from build123d import *

# Parameters (mm, degrees)
F0_W     = 70
F0_H     = 70
F1_DEPTH = 10
F2_R     = 10
F3_T     = -2.5
F4_W     = 13
F4_H     = 28.6
F4_R     = 11
F4_R_2   = 9.5
F5_DEPTH = 25


with BuildPart() as f1:
    # F0 (on Top) → F1 (new body)
    with BuildSketch(Plane.XY):
        with Locations((0, 1.327967)):
            Rectangle(F0_W, F0_H)
    extrude(amount=F1_DEPTH)

    # F2
    f2_edges = [f1.edges().sort_by_distance(p)[0] for p in [
        (35, 36.327967, 5),
        (35, -33.672033, 5),
        (-35, 36.327967, 5),
        (-35, -33.672033, 5),
    ]]
    fillet(f2_edges, radius=F2_R)

    # F3
    f3_openings = [f1.faces().sort_by_distance(p)[0] for p in [
        (0, 1.327967, 10),
    ]]
    offset(amount=F3_T, openings=f3_openings)

    # F4 (on face) → F5 (cut)
    with BuildSketch(Plane(origin=(0, 0, 0), x_dir=(1, 0, 0), z_dir=(0, 0, -1))):
        with Locations((17, 0)):
            Rectangle(F4_W, F4_H)
        with Locations((-16, -17.5)):
            Circle(F4_R)
        with Locations((-16, 17.5)):
            Circle(F4_R_2)
    extrude(amount=-F5_DEPTH, mode=Mode.SUBTRACT)


solid = f1.part
Could you check a few things on this model? Use its own coordinates, in mm. A direction names the side the tool comes from. Coordinates: 2 decimals unless noted, no trailing zeros. Loops run counter-clockwise (first coordinate to the right, second up) from the corner with the lowest first, then second, coordinate; pieces in that order, holes last.
1. Imagine slicing it at A-A (y = 17.5). Please give me the cut outline in (x, z), and give its area (4 significant figures).
2. We'd pull the mould along Y, two halves only. Please class faces 1 (the face through (0, 36.328, 5)), 2 (the face through (-32.148, -30.665, 5.07)), 3 (the face through (-18.059, -8.226, 1.232)), 4 (the face through (-35, 1, 5)): released by +Y, released by -Y, zero draft, split by the parting line, or undercut.
3. Imagine slicing it at B-B (x = -16). Please give me the cut outline in (y, z).
4. I need wall thicknesses on L1, parallel to Y at x = -16, z = 0.5; L2, parallel to X at y = -20, z = 7.5; L3, parallel to X at y = -17.5, z = 0.5. Which ranges of each line are inside material? Lowest first, please.
5. Imagine slicing it at C-C (z = 4.25). Please give me the cut outline in (x, y).
6. For faces 5 (the face through (0, 2, 0)), 6 (the face through (30.361, 31.573, 6.302)), 7 (the face through (10.5, 0, 1)), which set-ups out of +Z, -Z, +X, -X, +Y, -Y let a thin tool reach every point of the face, with its end or its side?
7. Imagine slicing it at D-D (x = 22.5). Please give me the cut outline in (y, z), and give its area (3 significant figures).
Computed values:
1. outline: (-35, 0) - (-27, 0) - (-27, 2.5) - (-32.5, 2.5) - (-32.5, 10) - (-35, 10) - close; (-5, 0) - (35, 0) - (35, 10) - (32.5, 10) - (32.5, 2.5) - (-5, 2.5) - close
1. area: 157.5 mm2
2. face 1: released by +Y
2. face 2: released by -Y
2. face 3: undercut
2. face 4: zero draft
3. outline: (-33.67, 0) - (-27, 0) - (-27, 2.5) - (-31.17, 2.5) - (-31.17, 10) - (-33.67, 10) - close; (-8, 0) - (6.5, 0) - (6.5, 2.5) - (-8, 2.5) - close; (28.5, 0) - (36.33, 0) - (36.33, 10) - (33.83, 10) - (33.83, 2.5) - (28.5, 2.5) - close
4. L1: y = -33.67 to -27, -8 to 6.5, 28.5 to 36.33
4. L2: x = -35 to -32.5, 32.5 to 35
4. L3: x = -35 to -25.5, -6.5 to 35
5. outline: (-35, -23.67) arc R10 ccw to (-25, -33.67) - (25, -33.67) arc R10 ccw to (35, -23.67) - (35, 26.33) arc R10 ccw to (25, 36.33) - (-25, 36.33) arc R10 ccw to (-35, 26.33) - close; hole (-32.5, -23.67) arc R7.5 ccw to (-25, -31.17) - (25, -31.17) arc R7.5 ccw to (32.5, -23.67) - (32.5, 26.33) arc R7.5 ccw to (25, 33.83) - (-25, 33.83) arc R7.5 ccw to (-32.5, 26.33) - close
6. face 5: -Z, +X, -X, +Y, -Y
6. face 6: +Z
6. face 7: +Z, -Z
7. outline: (-33.67, 0) - (-14.3, 0) - (-14.3, 2.5) - (-31.17, 2.5) - (-31.17, 10) - (-33.67, 10) - close; (14.3, 0) - (36.33, 0) - (36.33, 10) - (33.83, 10) - (33.83, 2.5) - (14.3, 2.5) - close
7. area: 141 mm2
